Check sheet for the modelled part. Datum: model origin and axes. Units: mm. A direction names the side the tool comes from. Give positions to 0.01 mm unless a question says otherwise; leave off trailing zeros. Order: outer loops, then holes, each group sorted by start corner. A loop starts at its lowest first (then second) coordinate and runs counter-clockwise, first axis right, second up.
from build123d import *

# Parameters (mm, degrees)
SKETCH1_W               = 38.1
SKETCH1_H               = 43.18
SKETCH1_R               = 1.905
BOSS_EXTRUDE1_DEPTH     = 1.5875
SKETCH2_W               = 2
SKETCH2_H               = 10.5378
BOSS_EXTRUDE2_DEPTH     = 38.1
SKETCH4_R               = 2.58285
CUT_EXTRUDE1_DEPTH      = 19.44
CUT_EXTRUDE1_DEPTH_BACK = 25.74
FILLET1_R               = 2.54
FILLET2_R               = 2.54
FILLET4_R               = 2.54
FILLET5_R               = 0.635


with BuildPart() as part:
    # Sketch1 → Boss-Extrude1 (new body)
    with BuildSketch(Plane(origin=(0, 0, 0), x_dir=(1, 0, 0), z_dir=(0, 1, 0))):
        with Locations((-19.05, 21.59)):
            Rectangle(SKETCH1_W, SKETCH1_H)
        with Locations((-33.02, 39.37)):
            Circle(SKETCH1_R, mode=Mode.SUBTRACT)
        with Locations((-33.02, 3.81)):
            Circle(SKETCH1_R, mode=Mode.SUBTRACT)
        with Locations((-5.08, 3.81)):
            Circle(SKETCH1_R, mode=Mode.SUBTRACT)
        with Locations((-5.08, 39.37)):
            Circle(SKETCH1_R, mode=Mode.SUBTRACT)
    extrude(amount=BOSS_EXTRUDE1_DEPTH)

    # Sketch2 → Boss-Extrude2 (add)
    with BuildSketch(Plane.ZY.offset(38.1)):
        with Locations((-23.74, 6.8564)):
            Rectangle(SKETCH2_W, SKETCH2_H)
        with Locations((-19.44, 6.8564)):
            Rectangle(SKETCH2_W, SKETCH2_H)
    extrude(amount=-BOSS_EXTRUDE2_DEPTH)

    # Sketch4 → Cut-Extrude1 (cut, two sides)
    with BuildSketch(Plane.XY.offset(-18.44)) as cut_extrude1_sk:
        with Locations((-34.29, 7.0453)):
            Circle(SKETCH4_R)
        with Locations((-19.05, 7.0453)):
            Circle(SKETCH4_R)
        with Locations((-3.81, 7.0453)):
            Circle(SKETCH4_R)
    extrude(amount=CUT_EXTRUDE1_DEPTH, mode=Mode.SUBTRACT)
    extrude(cut_extrude1_sk.sketch, amount=-CUT_EXTRUDE1_DEPTH_BACK, mode=Mode.SUBTRACT)

    # Fillet1
    fillet1_edges = [part.edges().sort_by_distance(p)[0] for p in [
        (0, 12.1253, -19.44),
        (-38.1, 12.1253, -19.44),
        (0, 12.1253, -23.74),
        (-38.1, 12.1253, -23.74),
    ]]
    fillet(fillet1_edges, radius=FILLET1_R)

    # Fillet2
    fillet2_edges = [part.edges().sort_by_distance(p)[0] for p in [
        (-19.05, 1.5875, -18.44),
        (-19.05, 1.5875, -24.74),
    ]]
    fillet(fillet2_edges, radius=FILLET2_R)

    # Fillet4
    fillet4_edges = [part.edges().sort_by_distance(p)[0] for p in [
        (0, 0.79375, 0),
        (-38.1, 0.79375, 0),
        (-38.1, 0.79375, -43.18),
        (0, 0.79375, -43.18),
    ]]
    fillet(fillet4_edges, radius=FILLET4_R)

    # Fillet5
    fillet5_edges = [part.edges().sort_by_distance(p)[0] for p in [
        (-38.1, 5.5864, -20.44),
        (0, 5.5864, -22.74),
        (-19.05, 12.1253, -22.74),
        (0, 5.5864, -20.44),
        (-38.1, 5.5864, -22.74),
        (-37.356051224, 11.381351224, -22.74),
        (-0.743948776, 11.381351224, -22.74),
        (-19.05, 12.1253, -20.44),
        (-37.356051224, 11.381351224, -20.44),
        (-0.743948776, 11.381351224, -20.44),
    ]]
    fillet(fillet5_edges, radius=FILLET5_R)


solid = part.part
1) Section check B-B, the plane x = -33.02. State how many separate pieces and enclosed holes the cut face has, then the cut area to 3 significant figures.
Recorded:
separate pieces: 5
enclosed holes: 0
area: 83.2 mm2
2) Section check D-D, the plane x = -12. Record the cut outline in (y, z) (1 decimal).
Recorded:
outline: (0, -43.2) - (1.6, -43.2) - (1.6, -27.3) arc R2.5 cw to (4.1, -24.7) - (12.1, -24.7) - (12.1, -23.4) arc R0.6 ccw to (11.5, -22.7) - (1.6, -22.7) - (1.6, -20.4) - (11.5, -20.4) arc R0.6 ccw to (12.1, -19.8) - (12.1, -18.4) - (4.1, -18.4) arc R2.5 cw to (1.6, -15.9) - (1.6, 0) - (0, 0) - close
3) Section check A-A, the plane z = -3.81. Record the cut outline in (x, y) (1 decimal), then the cut area to 3 significant figures.
Recorded:
outline: (-38.1, 0) - (-34.9, 0) - (-34.9, 1.6) - (-38.1, 1.6) - close; (-31.1, 0) - (-7, 0) - (-7, 1.6) - (-31.1, 1.6) - close; (-3.2, 0) - (0, 0) - (0, 1.6) - (-3.2, 1.6) - close
area: 48.4 mm2
4) Depth check by flat-ended pin: pin 1 Ø4.5 at (x, y) = (-3.81, 7.05) entering from +Z; pin 2 Ø5 at (x, z) = (-33.02, -3.81) entering from +Y; pin 3 Ø4 at (x, y) = (-31.5, 9.5) entering from -Z; pin 4 Ø2 at (y, z) = (6, -22) entering from -X. Enter the tip coordinate at first touch or a pass-through.
Recorded:
pin 1: passes through
pin 2: stops at y = 1.59
pin 3: stops at z = -24.74
pin 4: stops at x = -37.98
5) Draft check along X on faces 1 (the face through (-16.664, 6.056, -19.426)), 2 (the face through (-4.146, 9.606, -19.426)), 3 (the face through (-37.376, 11.361, -24.048)), 4 (the face through (-19, 1.588, -35)). Enter one of: +X half, -X half, draft (parallel to the pull), parting line (faces both ways), or undercut.
Recorded:
face 1: undercut
face 2: undercut
face 3: -X half
face 4: draft
6) Material ranges on L1, parallel to Z at x = -33.02, y = 1.1 (3 decimals); L2, parallel to X at y = 0.5, z = -39.37 (3 decimals); L3, parallel to Y at x = -3.81, z = -19.4, recorded low to high.
Recorded:
L1: z = -43.18 to -41.275, -37.465 to -5.715, -1.905 to 0
L2: x = -38.1 to -34.925, -31.115 to -6.985, -3.175 to 0
L3: y = 0 to 4.46, 9.63 to 12.13
7) Set-up check for faces 5 (the face through (-0.76, 11.4, -19.11)), 6 (the face through (-19, 10, -24.74)): record each of +Z, -Z, +X, -X, +Y, -Y from which the full face is reachable in a straight line by a thin tool's end or side.
Recorded:
face 5: +Z, -Z, +X, +Y
face 6: -Z, +X, -X, +Y
